Build history of the part. All positions in model axes, mm. Give positions to 0.01 mm unless a question says otherwise; leave off trailing zeros. Loops run counter-clockwise (first coordinate to the right, second up) from the corner with the lowest first, then second, coordinate; pieces in that order, holes last.
1) Band-saw the part on B-B on z = 37.25. List the corners of the cut face in (x, y), then the cut area to 3 significant figures.
2) Band-saw the part on C-C on z = 31.75. List the corners of the cut face in (x, y).
3) Band-saw the part on A-A on z = 36. List the corners of the cut face in (x, y).
4) Flat gauge pin, fed straight in: P1, Ø2, axis at x = -1, z = 36, coming from the +Y side. Where does the tip first touch, or does it go through?
5) Wall check: line 1 (Y direction, x = 2.25, z = 31.75); line 2 (Z direction, x = 1.5, y = 6.25); line 3 (Z direction, x = 9, y = 3). Give the ranges that are in metal, low to high.
```python
from build123d import *

# Parameters (mm, degrees)
F3_DEPTH       = 5
F3_DEPTH_BACK  = 50
F4_DEPTH       = 30
F7_DEPTH       = 5
F7_DEPTH_BACK  = 5
F10_DEPTH      = 5
F10_DEPTH_BACK = 5
F12_DEPTH      = 20


# Not quite as in the source:
# - a feature names something its author has since deleted; it is built from what else it names


with BuildPart() as f1:
    # F0 (on Front) → F1 (revolve)
    with BuildSketch(Plane.XZ):
        Polygon((0, 37.5), (0, 30), (10, 30), align=None)
    revolve(axis=Axis((0, 0, 33.75), (0, 0, 1)))

    # F2 (on Top) → F3 (cut, two sides)
    with BuildSketch(Plane.XY) as f3_sk:
        with BuildLine():
            Line((-6.644110661, 4.455984013), (-6.644110661, 7.4998452328))
            Line((-6.644110661, 7.4998452328), (-11.5474741906, 7.4998452328))
            Line((-11.5474741906, 7.4998452328), (-11.5474741906, -9.0728485957))
            Line((-11.5474741906, -9.0728485957), (-6.644110661, -9.0728485957))
            Line((-6.644110661, -9.0728485957), (-6.644110661, -4.455984013))
            ThreePointArc((-6.644110661, -4.455984013), (-8, 0), (-6.644110661, 4.455984013))
        make_face()
        with BuildLine():
            Line((-6.644110661, -4.455984013), (-6.644110661, 4.455984013))
            ThreePointArc((-6.644110661, 4.455984013), (-8, 0), (-6.644110661, -4.455984013))
        make_face()
    extrude(amount=-F3_DEPTH, mode=Mode.SUBTRACT)
    extrude(f3_sk.sketch, amount=F3_DEPTH_BACK, mode=Mode.SUBTRACT)

    # F2 (on Top) → F4 (cut)
    with BuildSketch(Plane.XY):
        with BuildLine():
            ThreePointArc((8, 0), (2.3288532277, 7.6535248509), (-6.644110661, 4.455984013))
            Line((-6.644110661, 4.455984013), (-6.644110661, -4.455984013))
            ThreePointArc((-6.644110661, -4.455984013), (2.3288532277, -7.6535248509), (8, 0))
        make_face()
    extrude(amount=F4_DEPTH, mode=Mode.SUBTRACT)

    # F6 (on line) → F7 (cut, two sides)
    with BuildSketch(Plane(origin=(3.1843009926, -8.1633897791, 0), x_dir=(-0.9316321862, -0.3634026275, 0), z_dir=(-0.3634026275, 0.9316321862, 0))) as f7_sk:
        with BuildLine():
            ThreePointArc((0, 28), (-4.026334039, 15), (0, 2))
            ThreePointArc((0, 2), (4.026334039, 15), (0, 28))
        make_face()
    extrude(amount=F7_DEPTH, mode=Mode.SUBTRACT)
    extrude(f7_sk.sketch, amount=-F7_DEPTH_BACK, mode=Mode.SUBTRACT)

    # F9 (on line) → F10 (cut, two sides)
    with BuildSketch(Plane(origin=(3.1843009926, 8.1633897791, 0), x_dir=(0.9316321862, -0.3634026275, 0), z_dir=(-0.3634026275, -0.9316321862, 0))) as f10_sk:
        with BuildLine():
            ThreePointArc((0, 28), (-4.026334039, 15), (0, 2))
            ThreePointArc((0, 2), (4.026334039, 15), (0, 28))
        make_face()
    extrude(amount=-F10_DEPTH, mode=Mode.SUBTRACT)
    extrude(f10_sk.sketch, amount=F10_DEPTH_BACK, mode=Mode.SUBTRACT)

    # F11 (on Right) → F12 (cut)
    with BuildSketch(Plane.YZ):
        with BuildLine():
            ThreePointArc((0, 28), (-4.026334039, 15), (0, 2))
            ThreePointArc((0, 2), (4.026334039, 15), (0, 28))
        make_face()
    extrude(amount=F12_DEPTH, mode=Mode.SUBTRACT)


solid = f1.part
```
Findings below:
1. outline: circle Ø0.67 at (0, 0)
1. area: 0.349 mm2
2. outline: (-6.64, -3.83) arc R7.67 ccw (long way) to (-6.64, 3.83) - close
3. outline: circle Ø4 at (0, 0)
4. P1: stops at y = 3.21
5. line 1: y = -7.33 to 7.33
5. line 2: z = 30 to 32.68
5. line 3: z = 30 to 30.38
